```python
from build123d import *

# Parameters (mm, degrees)
SKETCH1_R           = 5
BOSS_EXTRUDE1_DEPTH = 10
SKETCH2_R           = 8
BOSS_EXTRUDE2_DEPTH = 7
SKETCH3_R           = 4
BOSS_EXTRUDE3_DEPTH = 21
CHAMFER1_SIZE       = 2


with BuildPart() as part:
    # Sketch1 → Boss-Extrude1 (new body)
    with BuildSketch(Plane(origin=(0, 0, 0), x_dir=(1, 0, 0), z_dir=(0, 1, 0))):
        with Locations(Location((0, 0, 0), (0, 0, 270))):
            Circle(SKETCH1_R)
    extrude(amount=BOSS_EXTRUDE1_DEPTH)

    # Sketch2 → Boss-Extrude2 (add, symmetric)
    with BuildSketch(Plane(origin=(0, 0, 0), x_dir=(0, 0, -1), z_dir=(1, 0, 0))):
        with Locations((0, 13)):
            Circle(SKETCH2_R)
    extrude(amount=BOSS_EXTRUDE2_DEPTH, both=True)

    # Sketch3 → Boss-Extrude3 (add, symmetric)
    with BuildSketch(Plane.XY):
        with Locations(Location((0, 14.305369128, 0), (0, 0, 180))):
            Circle(SKETCH3_R)
    extrude(amount=BOSS_EXTRUDE3_DEPTH, both=True)

    # Chamfer1
    chamfer1_edges = [part.edges().sort_by_distance(p)[0] for p in [
        (-7, 13, 8),
        (7, 13, 8),
    ]]
    chamfer(chamfer1_edges, length=CHAMFER1_SIZE - 0.0001)  # a hair under: the kernel refuses the full size


solid = part.part
```
For this review, take the finished solid that the model builds, in its own axes (mm). A direction names the side the tool comes from. Give positions to 0.01 mm unless a question says otherwise; leave off trailing zeros. Write each loop counter-clockwise with the first axis right and the second up, starting at its lowest first coordinate (ties: lowest second). Pieces come first, ordered by that corner, then holes.
Item 1: Insertion check: P1, Ø6, axis at x = 0.5, z = -4.5, coming from the +Y side; P2, Ø4, axis at x = -1, z = 5.5, coming from the +Y side; P3, Ø8, axis at y = 14, z = 13, coming from the +X side. Each pin has a flat end and moves straight along its axis. Give the tip position at first contact, or say it passes through.
Item 2: Machinability: for faces 1 (the face through (1.5, 2.58, 4.77)), 2 (the face through (0.87, 18.21, 13.6)), 3 (the face through (0.87, 18.21, -13.39)), which of the approach directions +Z, -Z, +X, -X, +Y, -Y give a long, thin tool a straight path to every point of the face, cutting with its end or side? Answer none if there is none.
Item 3: Wall thickness on probe 1 along X at (y, z) = (14.25, 9.5); probe 2 along Y at (x, z) = (0, -12); probe 3 along Y at (x, z) = (-2.5, -2): over which ranges is each line inside the solid? List them lowest first.
Item 4: Take a section at C-C (y = 1.5). Give the boundary of the cut face in (x, z).
Item 5: Take a section at D-D (z = 15.5). Give the boundary of the cut face in (x, y), and give its area (3 significant figures).
Item 6: Take a section at B-B (x = 3). Give the boundary of the cut face in (y, z).
Established:
1. P1: stops at y = 20.86
1. P2: stops at y = 20.19
1. P3: stops at x = 4
2. face 1: -Y
2. face 2: +Z
2. face 3: -Z
3. probe 1: x = -4 to 4
3. probe 2: y = 10.31 to 18.31
3. probe 3: y = 0 to 20.75
4. outline: circle Ø10 at (0, 0)
5. outline: circle Ø8 at (0, 14.31)
5. area: 50.3 mm2
6. outline: (0, -4) - (6.07, -4) arc R8 ccw to (11.66, -7.89) - (11.66, -21) - (16.95, -21) - (16.95, -6.96) arc R8 ccw to (16.95, 6.96) - (16.95, 21) - (11.66, 21) - (11.66, 7.89) arc R8 ccw to (6.07, 4) - (0, 4) - close
